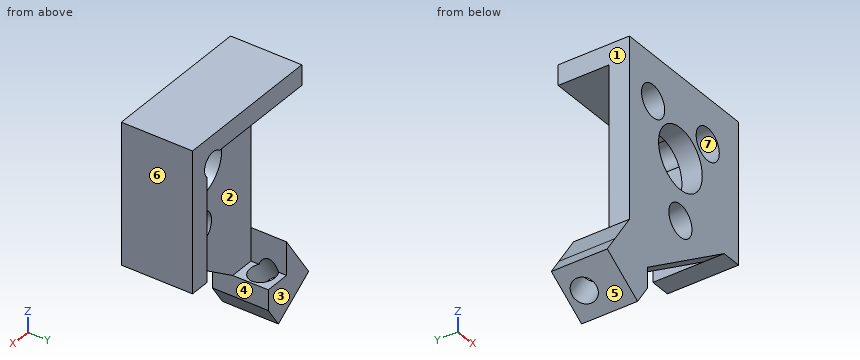
from build123d import *

# Parameters (mm, degrees)
SKETCH1_W                     = 8.5
SKETCH1_H                     = 11.5
BOSS_EXTRUDE1_DEPTH           = 3.5
SKETCH2_W                     = 6.5
SKETCH2_H                     = 9.5
CUT_EXTRUDE1_DEPTH            = 2.5
SKETCH3_R                     = 1.5
CUT_EXTRUDE2_DEPTH            = 2
SKETCH6_R                     = 0.5953125
CUT_EXTRUDE5_DEPTH            = 2.5
SKETCH7_R                     = 0.79375
CUT_EXTRUDE6_DEPTH            = 2
BOSS_EXTRUDE2_DEPTH           = 3.5
SKETCH14_W                    = 5.965258944
SKETCH14_H                    = 5.132960456
CUT_EXTRUDE8_DEPTH            = 0.75
TAP_DRILL_FOR_0_80_TAP1_D     = 1.19126
TAP_DRILL_FOR_0_80_TAP1_DEPTH = 7.11
TAP_DRILL_FOR_0_80_TAP1_TIP   = 0.357890611
CUT_EXTRUDE7_REACH            = 5.5


with BuildPart() as part:
    # Sketch1 → Boss-Extrude1 (new body)
    with BuildSketch(Plane(origin=(0, 0, 0), x_dir=(1, 0, 0), z_dir=(0, 1, 0))):
        Rectangle(SKETCH1_W, SKETCH1_H)
    extrude(amount=BOSS_EXTRUDE1_DEPTH)

    # Sketch2 → Cut-Extrude1 (cut)
    with BuildSketch(Plane(origin=(0, 3.5, 0), x_dir=(1, 0, 0), z_dir=(0, 1, 0))):
        Rectangle(SKETCH2_W, SKETCH2_H)
    extrude(amount=-CUT_EXTRUDE1_DEPTH, mode=Mode.SUBTRACT)

    # Sketch3 → Cut-Extrude2 (cut, through all)
    with BuildSketch(Plane(origin=(0, 1, 0), x_dir=(1, 0, 0), z_dir=(0, 1, 0))):
        with Locations((0.25, -1.75)):
            Circle(SKETCH3_R)
    extrude(amount=-CUT_EXTRUDE2_DEPTH, mode=Mode.SUBTRACT)

    # Sketch6 → Cut-Extrude5 (cut)
    with BuildSketch(Plane(origin=(0, 3.5, 0), x_dir=(1, 0, 0), z_dir=(0, 1, 0))):
        with Locations((2.829050494, -4.329050494)):
            Circle(SKETCH6_R)
    extrude(amount=-CUT_EXTRUDE5_DEPTH, mode=Mode.SUBTRACT)

    # Sketch7 → Cut-Extrude6 (cut, through all)
    with BuildSketch(Plane(origin=(0, 1, 0), x_dir=(1, 0, 0), z_dir=(0, 1, 0))):
        with Locations((0.25, 1.25)):
            Circle(SKETCH7_R)
        with Locations((-1.625, -3.5)):
            Circle(SKETCH7_R)
        with Locations((2.125, -3.5)):
            Circle(SKETCH7_R)
    extrude(amount=-CUT_EXTRUDE6_DEPTH, mode=Mode.SUBTRACT)

    # Sketch9 → Boss-Extrude2 (add)
    with BuildSketch(Plane(origin=(0, 3.5, 0), x_dir=(1, 0, 0), z_dir=(0, 1, 0))):
        Polygon((-2.69064642, 6.789569053), (-4.770772156, 5.402818562), (-4.001541387, 4.248972409), (-3.411634369, 4.642243754), (-2.511322669, 5.242451554), (-1.921415651, 5.635722899), align=None)
    extrude(amount=-BOSS_EXTRUDE2_DEPTH)

    # Sketch14 → Cut-Extrude8 (cut)
    with BuildSketch(Plane(origin=(0, 3.5, 0), x_dir=(1, 0, 0), z_dir=(0, 1, 0))):
        with Locations((-3.25, 4.75)):
            Rectangle(SKETCH14_W, SKETCH14_H)
    extrude(amount=-CUT_EXTRUDE8_DEPTH, mode=Mode.SUBTRACT)

    # Tap Drill for #0-80 Tap1
    with Locations(Plane(origin=(-3.961538462, 0, -5.942307692), x_dir=(-0.832050294, 0, 0.554700196), z_dir=(-0.554700196, 0, -0.832050294))):
        with Locations((-0.27742214, 1.875)):
            Hole(TAP_DRILL_FOR_0_80_TAP1_D / 2, depth=TAP_DRILL_FOR_0_80_TAP1_DEPTH)
            with Locations((0, 0, -(TAP_DRILL_FOR_0_80_TAP1_DEPTH + TAP_DRILL_FOR_0_80_TAP1_TIP / 2))):  # 118° drill point
                Cone(0, TAP_DRILL_FOR_0_80_TAP1_D / 2, TAP_DRILL_FOR_0_80_TAP1_TIP, mode=Mode.SUBTRACT)

    # Sketch13 → Cut-Extrude7 (cut, up to next)
    with BuildSketch(Plane(origin=(0, 3.5, 0), x_dir=(1, 0, 0), z_dir=(0, 1, 0)), mode=Mode.PRIVATE) as cut_extrude7_sk1:
        Polygon((-1.997600385, 5.75), (-1.997600385, 4.75), (3.25, 1.170806318), (4.25, 1.170806318), (4.25, 5.75), align=None)
    cut_extrude7_tool1 = extrude(cut_extrude7_sk1.sketch, amount=-CUT_EXTRUDE7_REACH, mode=Mode.PRIVATE) & part.part
    add(cut_extrude7_tool1.solids().sort_by_distance((1.797917, 3.5, -3.996239))[0], mode=Mode.SUBTRACT)
    # Sketch13 → Cut-Extrude7 (cut, up to next)
    with BuildSketch(Plane(origin=(0, 3.5, 0), x_dir=(1, 0, 0), z_dir=(0, 1, 0)), mode=Mode.PRIVATE) as cut_extrude7_sk2:
        Polygon((-4.25, 4.621660328), (-3.25, 3.121660328), (-3.25, -5.75), (-4.25, -5.75), align=None)
    cut_extrude7_tool2 = extrude(cut_extrude7_sk2.sketch, amount=-CUT_EXTRUDE7_REACH, mode=Mode.PRIVATE) & part.part
    add(cut_extrude7_tool2.solids().sort_by_distance((-3.762992, 3.5, 0.929426))[0], mode=Mode.SUBTRACT)


solid = part.part
Verification items for the finished model (mm, model axes). Face numbers are marked on the shaded views. A direction names the side the tool comes from. Coordinates: 2 decimals unless noted, no trailing zeros. Loops run counter-clockwise (first coordinate to the right, second up) from the corner with the lowest first, then second, coordinate; pieces in that order, holes last. Notation, with made-up numbers: (64.5, 89.25) -> (121.5, 89.25) arc R30 ccw to (121.5, 127.25) -> close; hole circle Ø2 at (78.25, 39). An arc over 180 degrees is marked (long way). Answer as CSV lines item,"result".
1) Cross-section at D-D, the plane z = -3.5. Record the cut outline in (x, y), then the cut area to 3 significant figures.
Found:
outline,"(-3.5, 0) -> (-0.16, 0) -> (-0.16, 1) -> (-3.25, 1) -> (-3.25, 2.75) -> (-3.5, 2.75) -> close"
area,"3.78 mm2"
2) Cross-section at B-B, the plane x = 0.75. Record the cut outline in (y, z).
Found:
outline,"(0, -2.88) -> (1, -2.88) -> (1, -1.87) -> (0, -1.87) -> close; (0, -0.63) -> (1, -0.63) -> (1, 0.34) -> (0, 0.34) -> close; (0, 3.16) -> (1, 3.16) -> (1, 4.75) -> (3.5, 4.75) -> (3.5, 5.75) -> (0, 5.75) -> close"
3) Depth check by flat-ended pin: pin 1 (4 mm diameter, centred on x = 1.5, z = 3.5, fed in from +Y); pin 2 (3.5 mm diameter, centred on x = -1, z = 0, fed in from +Y); pin 3 (1.1 mm diameter, centred on y = 1, z = -5.5, fed in from +X); pin 4 (3 mm diameter, centred on x = -3, z = -4.5, fed in from +Y). Enter the tip coordinate at first touch or a pass-through.
Found:
pin 1,"stops at y = 3.5"
pin 2,"stops at y = 1"
pin 3,"stops at x = -2"
pin 4,"stops at y = 2.75"
4) Tool access check on the marked faces 1, 2, 3 and 4. Record the directions out of +Z, -Z, +X, -X, +Y, -Y that give a thin tool (end or side, any length) a straight path to the whole face; none if there is none.
Found:
face 1,"+Z, -X, +Y, -Y"
face 2,"+Y"
face 3,"-Z, +X, -X, +Y"
face 4,"-Z, +X, +Y, -Y"
5) Cross-section at C-C, the plane x = 2. Record the cut outline in (y, z).
Found:
outline,"(0, -2.02) -> (1, -2.02) -> (1, 2.72) -> (0, 2.72) -> close; (0, 4.28) -> (1, 4.28) -> (1, 4.75) -> (3.5, 4.75) -> (3.5, 5.75) -> (0, 5.75) -> close"
6) Cross-section at A-A, the plane z = 1.75. Record the cut outline in (x, y).
Found:
outline,"(-3.25, 0) -> (-1.25, 0) -> (-1.25, 1) -> (-3.25, 1) -> close; (1.75, 0) -> (4.25, 0) -> (4.25, 3.5) -> (3.25, 3.5) -> (3.25, 1) -> (1.75, 1) -> close"
7) Thickness scan on L1, parallel to X at y = 0.2, z = 3.5; L2, parallel to Z at x = 0.25, y = 0.25; L3, parallel to Y at x = 2.75, z = 1.5. Record the ranges inside material, lowest first. Write a range as from..to.
Found:
L1,"x = -3.25..-2.42, -0.83..1.33, 2.92..4.25"
L2,"z = -3.22..-2.04, -0.46..0.25, 3.25..5.75"
L3,"y = 0..1"
8) Release check for a two-part mould opening along Z. For the marked faces 5, 6 and 7 record: +Z half, -Z half, draft (parallel to the pull), parting line (faces both ways), or undercut.
Found:
face 5,"-Z half"
face 6,"draft"
face 7,"undercut"
